Read the model definition and answer for the solid it produces. Units are mm, in the model's axes. Face numbers are marked on the shaded views. A direction names the side the tool comes from. Give positions to 0.01 mm unless a question says otherwise; leave off trailing zeros. Loops run counter-clockwise (first coordinate to the right, second up) from the corner with the lowest first, then second, coordinate; pieces in that order, holes last. Notation, with made-up numbers: (-9, 22.5) - (14, 22.5) arc R26 cw to (14, 44.5) - close; hole circle Ø10 at (-12, 44). An arc over 180 degrees is marked (long way). Put each result on its own line as item: value. Start each with the question number.
1. Consider L1, parallel to X at y = 10, z = 15.4; L2, parallel to X at y = 12.5, z = 10; L3, parallel to X at y = 10, z = 1.3. Determine where each line is inside the solid, lowest interval first. Write a range as from..to.
2. A cutting plane is placed at A-A, the plane x = 15. Determine the outline of the cut face in (y, z).
3. A cutting plane is placed at B-B, the plane z = 10. Determine the outline of the cut face in (x, y).
4. For a pull along X with two mould halves and no side action, classify the marked faces 1, 2, 3 and 4 as released by +X, released by -X, zero draft, split by the parting line, or undercut.
5. Given pin 1 Ø8 at (y, z) = (8.5, 4.5) entering from -X; pin 2 Ø10 at (x, z) = (28, 11) entering from +Y; pin 3 Ø1.5 at (x, y) = (-1.5, 4) entering from +Z; pin 4 Ø4 at (x, y) = (47.17, 10) entering from -Z, each flat-ended and moving along its own axis, determine where each tip first touches the part or whether it passes through.
6. For the marked faces 5, 6 and 7, determine the directions among +Z, -Z, +X, -X, +Y, -Y from which every point of the face is accessible in a straight line to the end or side of a thin tool.
7. A cutting plane is placed at D-D, the plane x = -42.5. Determine the outline of the cut face in (y, z), plus the area to 3 significant figures.
8. A cutting plane is placed at C-C, the plane y = 4.5. Determine the outline of the cut face in (x, z).
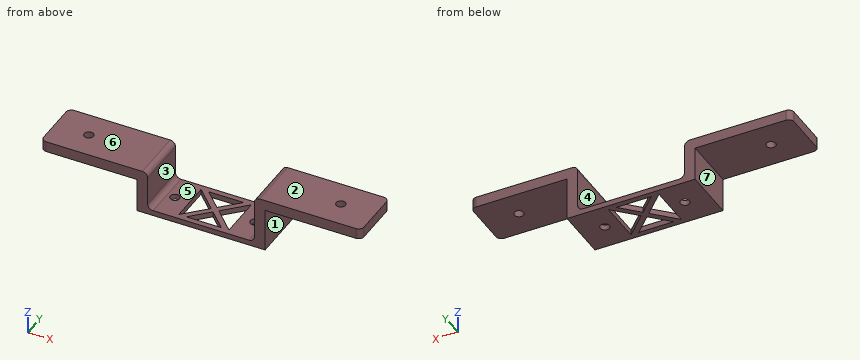
Autodesk Inventor part; units mm, degrees
ref_plane "YZ Plane" through (0, 0, 0) normal (1, 0, 0) x (0, 1, 0)
ref_plane "XZ Plane" through (0, 0, 0) normal (0, 1, 0) x (-1, 0, 0)
ref_plane "XY Plane" through (0, 0, 0) normal (0, 0, 1) x (1, 0, 0)
sketch "スケッチ1" plane through (0, 0, 0) normal (0, 1, 0) x (-1, 0, 0)
  line L0 (0, 20.7547) -> (0, -42.4528)
  line L1 (60, 16.75) -> (20, 16.75)
  line L2 (20, 16.75) -> (20, 2)
  line L3 (20, 2) -> (0, 2)
  line L4 (60, 16.75) -> (60, 12.75)
  line L5 (60, 12.75) -> (24, 12.75)
  line L6 (24, 12.75) -> (24, 0)
  line L7 (24, 0) -> (0, 0)
  line L8 (-20, 2) -> (0, 2)
  line L9 (-24, 0) -> (0, 0)
  line L10 (-24, 0) -> (-24, 16.25)
  line L11 (-24, 16.25) -> (-60, 16.25)
  line L12 (-60, 16.25) -> (-60, 20.25)
  line L13 (-60, 20.25) -> (-20, 20.25)
  line L14 (-20, 20.25) -> (-20, 2)
  dimension "d0" = 40
  dimension "d1" = 4
  dimension "d2" = 36
  dimension "d4" = 2
  dimension "d5" = 40
  dimension "d20" = 12.75
  dimension "d21" = 16.25
  dimension "d22" = 4
  dimension "d23" = 40
  dimension "d24" = 4
extrude "押し出し1" add sketch "スケッチ1" along normal blind 20
sketch "スケッチ2" plane through (24, 0, 0) normal (0, 0, -1) x (-1, 0, 0)
  line L0 (0, 10) -> (48, 10)
  line L1 (48, 0) -> (48, 20)
  line L2 (24, 0) -> (24, 20)
  line L3 (0, 20) -> (48, 20)
  circle A0 centre (9, 10) radius 1.75
  line L4 (14.5858, 18) -> (14.5858, 2)
  line L5 (14.5858, 2) -> (30.5858, 2)
  line L6 (30.5858, 2) -> (14.5858, 18)
  circle A1 centre (39, 10) radius 1.75
  line L7 (33.4142, 18) -> (33.4142, 2)
  line L8 (33.4142, 18) -> (17.4142, 18)
  line L9 (17.4142, 18) -> (33.4142, 2)
  line L10 (33.4142, 18) -> (17.4142, 2)
  line L11 (14.5858, 2) -> (30.5858, 18)
  point P0 (25.4142, 10)
  point P1 (24, 8.5858)
  point P2 (22.5858, 10)
  point P3 (24, 11.4142)
  dimension "d8" = 16
  dimension "d9" = 3.5
  dimension "d11" = 30
  dimension "d19" = 2
  dimension "d27" = 2
extrude "押し出し2" cut sketch "スケッチ2" against normal through all contours A1 L0 | L0 A1 | A0 L0 | L0 A0 | L7 L9 L0 | L0 L10 L7 | L8 L11 L2 | L2 L9 L8 | L6 L5 L2 | L2 L5 L10 | L11 L4 L0 | L0 L4 L6
sketch "スケッチ3" plane through (20, 0, 16.25) normal (0, 0, 1) x (1, 0, 0)
  line L0 (-80, 0) -> (-80, 20)
  line L1 (-80, 10) -> (40, 10)
  circle A0 centre (27.1661, 10) radius 1.75
  circle A1 centre (-67.25, 10) radius 1.75
  line L2 (40, 0) -> (40, 20)
  point P0 (-20, 0)
  dimension "d14" = 3.5
  dimension "d16" = 12.75
extrude "押し出し3" cut sketch "スケッチ3" along normal through all both and the other way through all
fillet "フィレット1" radius 2 4 edges at (60, 20, 18.25) (60, 0, 18.25) (-60, 20, 14.75) (-60, 0, 14.75)
fillet "フィレット2" radius 2 4 edges at (-20, 10, 16.75) (-20, 10, 2) (20, 10, 2) (20, 10, 20.25)
properties part number "joint2_sup"
Return value:
1. L1: x = -60..-49, -45.5..-20.11, 20..24
1. L2: x = -24..-20, 20..24
1. L3: x = -24..-16.75, -13.25..-9.41, -1.41..1.41, 9.41..13.25, 16.75..24
2. outline: (0, 0) - (8.25, 0) - (8.25, 2) - (0, 2) - close; (11.75, 0) - (20, 0) - (20, 2) - (11.75, 2) - close
3. outline: (-24, 0) - (-20, 0) - (-20, 20) - (-24, 20) - close; (20, 0) - (24, 0) - (24, 20) - (20, 20) - close
4. face 1: released by +X
4. face 2: zero draft
4. face 3: undercut
4. face 4: undercut
5. pin 1: stops at x = -24
5. pin 2: stops at y = 20
5. pin 3: passes through
5. pin 4: stops at z = 16.25
6. face 5: +Z, +Y, -Y
6. face 6: +Z, -X, +Y, -Y
6. face 7: -Z, -X, +Y, -Y
7. outline: (0, 12.75) - (20, 12.75) - (20, 16.75) - (0, 16.75) - close
7. area: 80.0 mm2
8. outline: (-60, 12.75) - (-24, 12.75) - (-24, 0) - (-9.41, 0) - (-9.41, 2) - (-18, 2) arc R2 cw to (-20, 4) - (-20, 14.75) arc R2 ccw to (-22, 16.75) - (-60, 16.75) - close; (-6.91, 0) - (-4.09, 0) - (-4.09, 2) - (-6.91, 2) - close; (4.09, 0) - (6.91, 0) - (6.91, 2) - (4.09, 2) - close; (9.41, 0) - (24, 0) - (24, 16.25) - (60, 16.25) - (60, 20.25) - (22, 20.25) arc R2 ccw to (20, 18.25) - (20, 4) arc R2 cw to (18, 2) - (9.41, 2) - close
